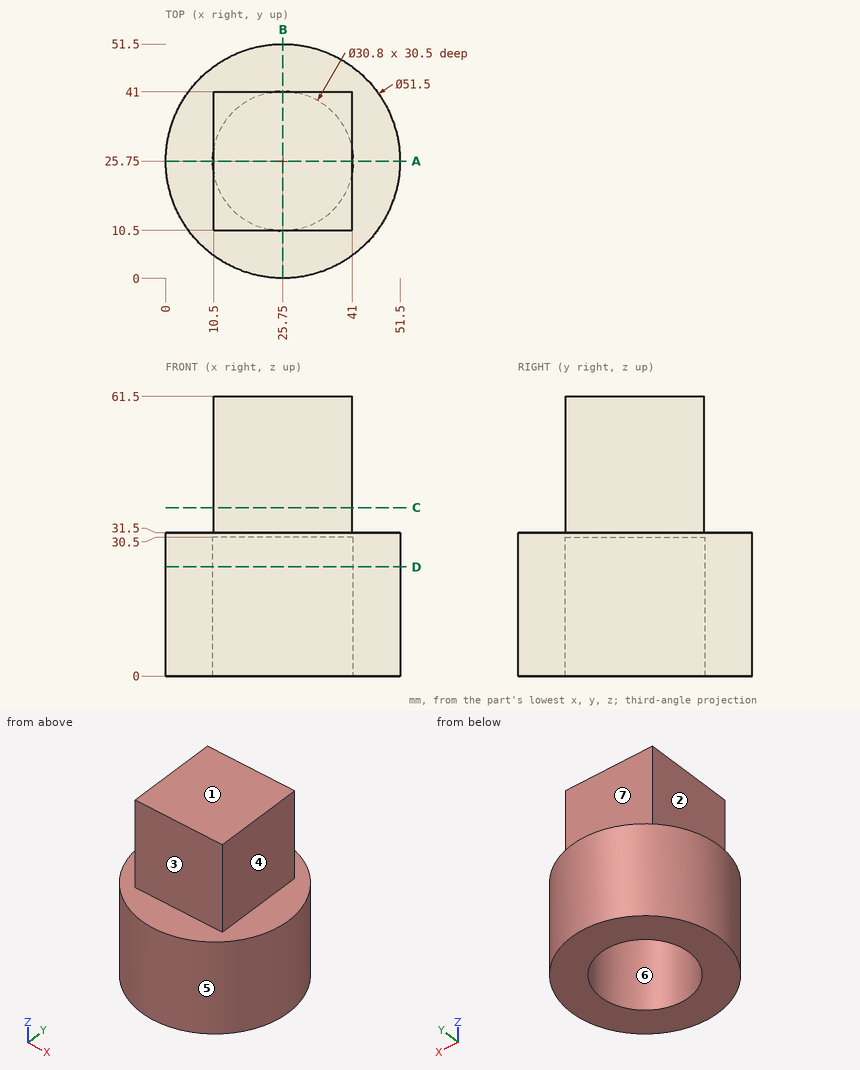
Answer from the drawing. Dimensions are ordinates in mm from the lowest x, y and z of the part. A direction names the side the tool comes from. Round coordinates to 2 decimals unless told otherwise and drop trailing zeros. Loops run counter-clockwise (first coordinate to the right, second up) from the corner with the lowest first, then second, coordinate; pieces in that order, holes last.
(1) The mould has two halves that part along X. Classify the marked faces 5, 6 and 7: pulls with the +X half, pulls with the -X half, needs draft (parallel to the pull), parting line crosses it, or undercut.
Computed values:
face 5: parting line crosses it
face 6: undercut
face 7: needs draft
(2) The part is cut by section D-D, the plane z = 24. Give the vertices of the cut face in (x, y), and give its area (3 significant figures).
Computed values:
outline: circle Ø51.5 at (25.75, 25.75); hole circle Ø30.8 at (25.75, 25.75)
area: 1,340 mm2
(3) Each of these flat-tipped pins is pushed along its axis until it touches: P1, Ø9, axis at y = 30, z = 41, coming from the -X side; P2, Ø5, axis at y = 34.5, z = 9, coming from the -X side; P3, Ø1, axis at x = 29, z = 12, coming from the +Y side; P4, Ø1.5, axis at y = 8, z = 49.5, coming from the +X side. Where does it stop, or does it pass through?
Computed values:
P1: stops at x = 10.5
P2: stops at x = 0.77
P3: stops at y = 51.35
P4: passes through
(4) Find the intervals of material crossed by L1, parallel to X at y = 25, z = 20; L2, parallel to Y at x = 39.5, z = 28, in increasing order.
Computed values:
L1: x = 0.01 to 10.37, 41.13 to 51.49
L2: y = 3.98 to 18.81, 32.69 to 47.52
(5) For the marked faces 1, 2, 3 and 4, determine the directions among +Z, -Z, +X, -X, +Y, -Y from which every point of the face is accessible in a straight line to the end or side of a thin tool.
Computed values:
face 1: +Z, +X, -X, +Y, -Y
face 2: +Z, -X, +Y, -Y
face 3: +Z, +X, -X, -Y
face 4: +Z, +X, +Y, -Y
(6) The part is cut by section A-A, the plane y = 25.75. Give the vertices of the cut face in (x, z).
Computed values:
outline: (0, 0) - (10.35, 0) - (10.35, 30.5) - (41.15, 30.5) - (41.15, 0) - (51.5, 0) - (51.5, 31.5) - (41, 31.5) - (41, 61.5) - (10.5, 61.5) - (10.5, 31.5) - (0, 31.5) - close
(7) The part is cut by section C-C, the plane z = 37. Give the vertices of the cut face in (x, y), and give its area (3 significant figures).
Computed values:
outline: (10.5, 10.5) - (41, 10.5) - (41, 41) - (10.5, 41) - close
area: 930 mm2
